```python
from build123d import *

# Parameters (mm, degrees)
F2_R     = 3.175
F5_DEPTH = 50.8
F3_R     = 0.51181
F6_DEPTH = 9.525
F4_R     = 0.51181
F7_DEPTH = 60.325


with BuildPart() as f5:
    # F2 (on Front) → F5 (new body)
    with BuildSketch(Plane.XZ):
        Circle(F2_R)
    extrude(amount=F5_DEPTH)

    # F3 (on Front) → F6 (join)
    with BuildSketch(Plane.XZ):
        Circle(F3_R)
    extrude(amount=-F6_DEPTH)

    # F4 (on Front) → F7 (join)
    with BuildSketch(Plane.XZ):
        Circle(F4_R)
    extrude(amount=F7_DEPTH)


solid = f5.part
```
Design review of the part built by this model. Coordinates are the model's own, in mm. Coordinates: 2 decimals unless noted, no trailing zeros. Order: outer loops, then holes, each group sorted by start corner. A loop starts at its lowest first (then second) coordinate and runs counter-clockwise, first axis right, second up. Notation, with made-up numbers: (11.25, 9) - (35.25, 9) arc R17 cw to (35.25, 30) - close; hole circle Ø1 at (37, 27.5). An arc over 180 degrees is marked (long way). Answer in a Markdown table with one row per item.
(1) Wall thickness on line 1 along Y through (x, z) = (2.5, 1); line 2 along X through (y, z) = (-10, 2); line 3 along X through (y, z) = (-5.5, 1.75): over which ranges is each line inside the solid? List them lowest first. Write a range as from..to.
Checked values:
| item | result |
|---|---|
| line 1 | -50.8..0 |
| line 2 | -2.47..2.47 |
| line 3 | -2.65..2.65 |
(2) Clearance check with a flat-ended pin moving along its axis: pin 1 (1 mm diameter, centred on y = -12, z = -2, fed in from +X). State where the tip first meets the part, or that it passes through.
Checked values:
| item | result |
|---|---|
| pin 1 | x = 2.8 |
(3) Consider section B-B on x = 2. State the section outline as (y, z) points.
Checked values:
| item | result |
|---|---|
| outline | (-50.8, -2.47) - (0, -2.47) - (0, 2.47) - (-50.8, 2.47) - close |
(4) Consider section D-D on y = -44. State the section outline as (x, z) points (3 decimals), plus the area to 3 significant figures.
Checked values:
| item | result |
|---|---|
| outline | circle Ø6.35 at (0, 0) |
| area | 31.7 mm^2 |
(5) Consider section A-A on y = 1.5. State the section outline as (x, z) points, plus the area to 3 significant figures.
Checked values:
| item | result |
|---|---|
| outline | circle Ø1.02 at (0, 0) |
| area | 0.823 mm^2 |
(6) Consider section C-C on z = 2. State the section outline as (x, y) points, plus the area to 3 significant figures.
Checked values:
| item | result |
|---|---|
| outline | (-2.47, -50.8) - (2.47, -50.8) - (2.47, 0) - (-2.47, 0) - close |
| area | 251 mm^2 |
